```python
from build123d import *

# Parameters (mm, degrees)
SKETCH1_W             = 93
SKETCH1_H             = 100
BOSS_EXTRUDE1_DEPTH   = 10
SKETCH7_W             = 70
SKETCH7_H             = 70
SKETCH7_W_2           = 50
SKETCH7_H_2           = 50
BOSS_EXTRUDE4_DEPTH   = 600
M5_TAPPED_HOLE1_D     = 4.2
M5_TAPPED_HOLE1_DEPTH = 12.4
M5_TAPPED_HOLE1_TIP   = 1.2618073
SKETCH11_R            = 2.75
CUT_EXTRUDE1_DEPTH    = 11
SKETCH12_R            = 5.5
CUT_EXTRUDE2_DEPTH    = 5.5


with BuildPart() as part:
    # Sketch1 → Boss-Extrude1 (new body)
    with BuildSketch(Plane(origin=(0, 0, 0), x_dir=(1, 0, 0), z_dir=(0, 1, 0))):
        Rectangle(SKETCH1_W, SKETCH1_H)
    extrude(amount=BOSS_EXTRUDE1_DEPTH)

    # Sketch7 → Boss-Extrude4 (add)
    with BuildSketch(Plane(origin=(0, 10, 0), x_dir=(1, 0, 0), z_dir=(0, 1, 0))):
        Rectangle(SKETCH7_W, SKETCH7_H)
        Rectangle(SKETCH7_W_2, SKETCH7_H_2, mode=Mode.SUBTRACT)
    extrude(amount=BOSS_EXTRUDE4_DEPTH)

    # M5 Tapped Hole1
    with Locations(Plane(origin=(0, 0, -35), x_dir=(-1, 0, 0), z_dir=(0, 0, -1))):
        with Locations((-20, 585), (20, 585), (20, 555), (-20, 555)):
            Hole(M5_TAPPED_HOLE1_D / 2, depth=M5_TAPPED_HOLE1_DEPTH)
            with Locations((0, 0, -(M5_TAPPED_HOLE1_DEPTH + M5_TAPPED_HOLE1_TIP / 2))):  # 118° drill point
                Cone(0, M5_TAPPED_HOLE1_D / 2, M5_TAPPED_HOLE1_TIP, mode=Mode.SUBTRACT)

    # Sketch11 → Cut-Extrude1 (cut, through all)
    with BuildSketch(Plane(origin=(0, 10, 0), x_dir=(1, 0, 0), z_dir=(0, 1, 0))):
        with Locations((-40, 40)):
            Circle(SKETCH11_R)
        with Locations((-40, -40)):
            Circle(SKETCH11_R)
        with Locations((40, -40)):
            Circle(SKETCH11_R)
        with Locations((40, 40)):
            Circle(SKETCH11_R)
    extrude(amount=-CUT_EXTRUDE1_DEPTH, mode=Mode.SUBTRACT)

    # Sketch12 → Cut-Extrude2 (cut)
    with BuildSketch(Plane(origin=(0, 10, 0), x_dir=(1, 0, 0), z_dir=(0, 1, 0))):
        with Locations((-40, 40)):
            Circle(SKETCH12_R)
        with Locations((40, 40)):
            Circle(SKETCH12_R)
        with Locations((40, -40)):
            Circle(SKETCH12_R)
        with Locations((-40, -40)):
            Circle(SKETCH12_R)
    extrude(amount=-CUT_EXTRUDE2_DEPTH, mode=Mode.SUBTRACT)


solid = part.part
```
CAD build for the part. Positions are in the model's coordinates, mm. A direction names the side the tool comes from. Round coordinates to 2 decimals unless told otherwise and drop trailing zeros. Loops run counter-clockwise (first coordinate to the right, second up) from the corner with the lowest first, then second, coordinate; pieces in that order, holes last. Notation, with made-up numbers: M 21,-5 L 31,-5 A32 cw 31,24 Z; hole C 30,69.25 d10. An arc over 180 degrees is marked long. Use a Markdown table: item, result. Add a question column.
(1) Cut at A-A (y = 390). Give the cut face in (x, z), and give its area (3 significant figures).
(2) Drill centre lines: line 1 (X direction, y = 6.9, z = 40); line 2 (Z direction, x = -40, y = 2.7); line 3 (Y direction, x = 20, z = -32). Where is each one in solid material? Low to high.
(3) Cut at B-B (z = -7). Give the cut face in (x, y), and give its area (3 significant figures).
(4) Flat gauge pins, fed straight in: pin 1 (12 mm diameter, centred on x = -42.5, z = -37.5, fed in from +Y); pin 2 (8 mm diameter, centred on y = 216.5, z = 4, fed in from -X); pin 3 (15 mm diameter, centred on y = 438.5, z = 3.5, fed in from +X); pin 4 (6.5 mm diameter, centred on x = 40, z = -40, fed in from -Y). Where does each tip first touch, or does it go through?
(5) Pull direction X, two halves, no side cores. Call faces 4 (the face through (-25, 306, 0)), 5 (the face through (-35, 306, 0)), 6 (the face through (-1, 5, -50)): +X half, -X half, draft (parallel to the pull), parting line (faces both ways), or undercut.
(6) Which spindle directions (+Z, -Z, +X, -X, +Y, -Y) get a long thin tool onto all of the face, cutting with end or side? Do faces 1 (the face through (-43, 4.5, 41)), 2 (the face through (35, 306, 0)), 3 (the face through (0, 306, -35)). Say none if no direction does.
Geometry says:
| question | item | result |
|---|---|---|
| 1 | outline | M -35,-35 L 35,-35 L 35,35 L -35,35 Z; hole M -25,-25 L 25,-25 L 25,25 L -25,25 Z |
| 1 | area | 2,400 mm² |
| 2 | line 1 | x = -46.5 to -45.5, -34.5 to 34.5, 45.5 to 46.5 |
| 2 | line 2 | z = -50 to -42.75, -37.25 to 37.25, 42.75 to 50 |
| 2 | line 3 | y = 0 to 552.9, 557.1 to 582.9, 587.1 to 610 |
| 3 | outline | M -46.5,0 L 46.5,0 L 46.5,10 L 35,10 L 35,610 L 25,610 L 25,10 L -25,10 L -25,610 L -35,610 L -35,10 L -46.5,10 Z |
| 3 | area | 12,900 mm² |
| 4 | pin 1 | stops at y = 10 |
| 4 | pin 2 | stops at x = -35 |
| 4 | pin 3 | stops at x = 35 |
| 4 | pin 4 | stops at y = 0 |
| 5 | face 4 | undercut |
| 5 | face 5 | -X half |
| 5 | face 6 | draft |
| 6 | face 1 | +Y |
| 6 | face 2 | +Z, -Z, +X, +Y |
| 6 | face 3 | -Z, +X, -X, +Y |
